Geometry: see drawing. Coordinates: mm, zero at the bounding-box minimum. A direction names the side the tool comes from. Coordinates: 2 decimals unless noted, no trailing zeros. Loops run counter-clockwise (first coordinate to the right, second up) from the corner with the lowest first, then second, coordinate; pieces in that order, holes last. Notation, with made-up numbers: (68.25, 69) -> (80.25, 69) arc R10 ccw to (80.25, 85) -> close; hole circle Ø11 at (5, 29). An arc over 180 degrees is marked (long way). One line per question, with ' | ' between items. Start each with the question number.
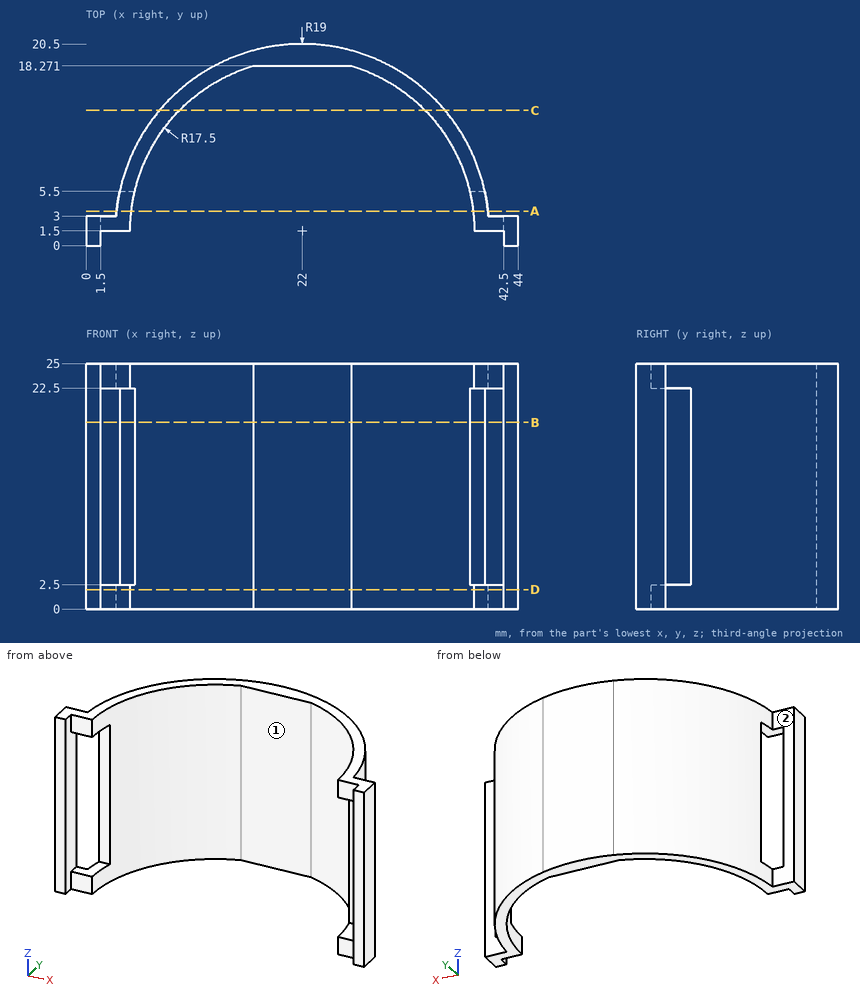
(1) Cut plane A-A, the plane y = 3.5. Return the cut outline in (x, z) (1 decimal).
(2) Cut plane D-D, the plane z = 2. Return the cut outline in (x, y).
(3) Cut plane B-B, the plane z = 19. Return the cut outline in (x, y) (1 decimal).
(4) Cut plane C-C, the plane y = 13.75. Return the cut outline in (x, z), and give its area (3 significant figures).
(5) Contact query for flat-ended pins moving along their axis: pin 1 Ø1.7 at (x, z) = (4, 17.5) entering from -Y; pin 2 Ø0.8 at (x, z) = (40.5, 24) entering from -Y; pin 3 Ø0.9 at (x, z) = (42, 18) entering from +Y; pin 4 Ø2.5 at (x, z) = (1.5, 16) entering from +Y. Output: stop coordinate, or through.
(6) Ray query, L1, parallel to X at y = 8.75, z = 3; L2, parallel to X at y = 4.25, z = 23.25; L3, parallel to Y at x = 22, z = 11. Return the intervals inside material, ascending.
(7) Access query for the marked faces 1 and 2. Directions: +Z, -Z, +X, -X, +Y, -Y. A direction counts if a zero-diameter tool reaches every point of the face in a straight line with its end or side. Return the directions, or none.
Here are the results:
1) outline: (3.1, 0) -> (4.6, 0) -> (4.6, 2.5) -> (3.1, 2.5) -> close; (3.1, 22.5) -> (4.6, 22.5) -> (4.6, 25) -> (3.1, 25) -> close; (39.4, 0) -> (40.9, 0) -> (40.9, 2.5) -> (39.4, 2.5) -> close; (39.4, 22.5) -> (40.9, 22.5) -> (40.9, 25) -> (39.4, 25) -> close
2) outline: (0, 0) -> (1.5, 0) -> (1.5, 1.5) -> (4.5, 1.5) arc R17.5 cw to (17, 18.27) -> (27, 18.27) arc R17.5 cw to (39.5, 1.5) -> (42.5, 1.5) -> (42.5, 0) -> (44, 0) -> (44, 3) -> (40.94, 3) arc R19 ccw to (27, 19.83) arc R19 ccw to (17, 19.83) arc R19 ccw to (3.06, 3) -> (0, 3) -> close
3) outline: (0, 0) -> (1.5, 0) -> (1.5, 3) -> (0, 3) -> close; (3.4, 5.5) -> (5, 5.5) arc R17.5 cw to (17, 18.3) -> (27, 18.3) arc R17.5 cw to (39, 5.5) -> (40.6, 5.5) arc R19 ccw to (27, 19.8) arc R19 ccw to (17, 19.8) arc R19 ccw to start; (42.5, 0) -> (44, 0) -> (44, 3) -> (42.5, 3) -> close
4) outline: (7.48, 0) -> (9.5, 0) -> (9.5, 25) -> (7.48, 25) -> close; (34.5, 0) -> (36.52, 0) -> (36.52, 25) -> (34.5, 25) -> close | area: 101 mm2
5) pin 1: stops at y = 5.5 | pin 2: stops at y = 1.5 | pin 3: passes through | pin 4: stops at y = 3
6) L1: x = 4.44 to 6.07, 37.93 to 39.56 | L2: x = 3.2 to 4.72, 39.28 to 40.8 | L3: y = 18.27 to 20.5
7) face 1: +Z, -Z, -Y | face 2: +Z, -Z, -X, +Y
